Part model, mm, in its own coordinate system. A direction names the side the tool comes from. Round coordinates to 2 decimals unless told otherwise and drop trailing zeros. Loops run counter-clockwise (first coordinate to the right, second up) from the corner with the lowest first, then second, coordinate; pieces in that order, holes last. Notation, with made-up numbers: (40.25, 40) -> (57.25, 40) arc R11 cw to (57.25, 56) -> close; hole circle Ø2 at (56, -19.75). An arc over 180 degrees is marked (long way). Answer as a JSON object with one key per item and string values. Group by question number.
Autodesk Inventor part; units mm, degrees
ref_plane "YZ Plane" through (0, 0, 0) normal (1, 0, 0) x (0, 1, 0)
ref_plane "XZ Plane" through (0, 0, 0) normal (0, 1, 0) x (-1, 0, 0)
ref_plane "XY Plane" through (0, 0, 0) normal (0, 0, 1) x (1, 0, 0)
sketch "Esquisse1" plane through (0, 0, 0) normal (0, 0, 1) x (1, 0, 0)
  line L0 (0, 0) -> (75, 0)
  line L1 (75, 0) -> (75, 75)
  line L2 (75, 75) -> (0, 75)
  line L3 (0, 75) -> (0, 0)
  dimension "d0" = 75
  dimension "d1" = 75
extrude "Extrusion1" add sketch "Esquisse1" along normal blind 2
sketch "Esquisse2" plane through (0, 0, 2) normal (0, 0, 1) x (1, 0, 0)
  line L0 (32, 36) -> (42, 36)
  line L1 (42, 36) -> (42, 39)
  line L2 (42, 39) -> (32, 39)
  line L3 (32, 39) -> (32, 36)
  line L4 (0, 0) -> (75, 0)
  line L5 (0, 75) -> (0, 0)
  dimension "d4" = 10
  dimension "d5" = 3
  dimension "d6" = 36
  dimension "d7" = 32
extrude "Extrusion2" cut sketch "Esquisse2" against normal blind 2
properties part number "Pièce-moteur-vis_CPY"
Item 1: Band-saw the part on A-A, the plane x = 38. List the corners of the cut face in (y, z).
Item 2: Two-plate mould, pull along X, no slides. Class faces 3 (the face through (37, 30, 0)), 4 (the face through (75, 37, 1)), 5 (the face through (42, 37, 1)), 6 (the face through (37, 39, 1)): pulls with the +X half, pulls with the -X half, needs draft (parallel to the pull), parting line crosses it, or undercut.
Item 3: Which spindle directions (+Z, -Z, +X, -X, +Y, -Y) get a long thin tool onto all of the face, cutting with end or side? Do faces 1 (the face through (37, 0, 1)), 2 (the face through (32, 38, 1)). Say none if no direction does.
Item 4: Drill centre lines: line 1 (Y direction, x = 37.5, z = 1.8); line 2 (X direction, y = 37.5, z = 1.8). Where is each one in solid material? Low to high.
Entries:
{
 "1": {"outline": "(0, 0) -> (36, 0) -> (36, 2) -> (0, 2) -> close; (39, 0) -> (75, 0) -> (75, 2) -> (39, 2) -> close"},
 "2": {"face 3": "needs draft", "face 4": "pulls with the +X half", "face 5": "undercut", "face 6": "undercut"},
 "3": {"face 1": "+Z, -Z, +X, -X, -Y", "face 2": "+Z, -Z"},
 "4": {"line 1": "0 to 36, 39 to 75", "line 2": "0 to 32, 42 to 75"}
}
